Build history of the part. All positions in model axes, mm. Face numbers are marked on the shaded views. Give positions to 0.01 mm unless a question says otherwise; leave off trailing zeros. Order: outer loops, then holes, each group sorted by start corner. A loop starts at its lowest first (then second) coordinate and runs counter-clockwise, first axis right, second up. Notation, with made-up numbers: M 59,71 L 96,71 A18 cw 96,100 Z; hole C -34,72 d10. An arc over 180 degrees is marked long. Answer as CSV lines item,"result".
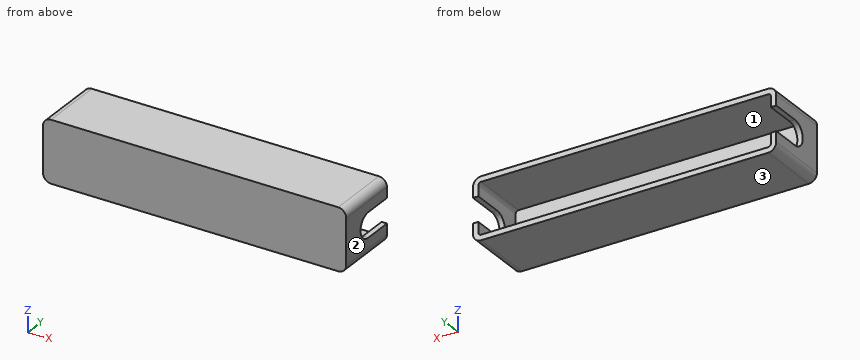
from build123d import *

# Parameters (mm, degrees)
BOSS_EXTRUDE1_DEPTH = 24
SHELL2_T            = -2
CUT_EXTRUDE1_DEPTH  = 117.091558694


with BuildPart() as part:
    # Sketch1 → Boss-Extrude1 (new body)
    with BuildSketch(Plane(origin=(0, 0, 0), x_dir=(1, 0, 0), z_dir=(0, 1, 0))):
        with BuildLine():
            Line((-53.5, -11.5), (53.5, -11.5))
            ThreePointArc((53.5, -11.5), (55.621320344, -10.621320344), (56.5, -8.5))
            Line((56.5, -8.5), (56.5, 8.5))
            ThreePointArc((56.5, 8.5), (55.621320344, 10.621320344), (53.5, 11.5))
            Line((53.5, 11.5), (-53.5, 11.5))
            ThreePointArc((-53.5, 11.5), (-55.621320344, 10.621320344), (-56.5, 8.5))
            Line((-56.5, 8.5), (-56.5, -8.5))
            ThreePointArc((-56.5, -8.5), (-55.621320344, -10.621320344), (-53.5, -11.5))
        make_face()
    extrude(amount=BOSS_EXTRUDE1_DEPTH)

    # Shell2
    shell2_openings = [part.faces().sort_by_distance(p)[0] for p in [
        (0, 24, 0),
    ]]
    offset(amount=SHELL2_T, openings=shell2_openings, kind=Kind.INTERSECTION)

    # Sketch4 → Cut-Extrude1 (cut, through all)
    with BuildSketch(Plane(origin=(56.5, 0, 0), x_dir=(0, 0, -1), z_dir=(1, 0, 0))):
        with BuildLine():
            Line((-4.588804417, 24), (-4.588804417, 13))
            ThreePointArc((-4.588804417, 13), (0, 8.411195583), (4.588804417, 13))
            Line((4.588804417, 13), (4.588804417, 24))
            Line((4.588804417, 24), (-4.588804417, 24))
        make_face()
    extrude(amount=-CUT_EXTRUDE1_DEPTH, mode=Mode.SUBTRACT)


solid = part.part
Item 1: Band-saw the part on A-A (y = 17). Give the cut face in (x, z).
Geometry says:
outline,"M -56.5,-8.5 A3 ccw -53.5,-11.5 L 53.5,-11.5 A3 ccw 56.5,-8.5 L 56.5,-4.59 L 54.5,-4.59 L 54.5,-8.5 A1 cw 53.5,-9.5 L -53.5,-9.5 A1 cw -54.5,-8.5 L -54.5,-4.59 L -56.5,-4.59 Z; M -56.5,4.59 L -54.5,4.59 L -54.5,8.5 A1 cw -53.5,9.5 L 53.5,9.5 A1 cw 54.5,8.5 L 54.5,4.59 L 56.5,4.59 L 56.5,8.5 A3 ccw 53.5,11.5 L -53.5,11.5 A3 ccw -56.5,8.5 Z"
Item 2: Band-saw the part on B-B (x = 14.5). Give the cut face in (y, z).
Geometry says:
outline,"M 0,-11.5 L 24,-11.5 L 24,-9.5 L 2,-9.5 L 2,9.5 L 24,9.5 L 24,11.5 L 0,11.5 Z"
Item 3: Band-saw the part on D-D (y = 10). Give the cut face in (x, z), and give its area (3 significant figures).
Geometry says:
outline,"M -56.5,-8.5 A3 ccw -53.5,-11.5 L 53.5,-11.5 A3 ccw 56.5,-8.5 L 56.5,-3.47 L 54.5,-3.47 L 54.5,-8.5 A1 cw 53.5,-9.5 L -53.5,-9.5 A1 cw -54.5,-8.5 L -54.5,-3.47 L -56.5,-3.47 Z; M -56.5,3.47 L -54.5,3.47 L -54.5,8.5 A1 cw -53.5,9.5 L 53.5,9.5 A1 cw 54.5,8.5 L 54.5,3.47 L 56.5,3.47 L 56.5,8.5 A3 ccw 53.5,11.5 L -53.5,11.5 A3 ccw -56.5,8.5 Z"
area,"493 mm2"
Item 4: Probe line 1 along X through (y, z) = (17, 7.25); line 2 along Z through (x, y) = (36, 13); line 3 along Y through (x, z) = (40.5, 8). List the from-to ranges inside material, lowest first. Write a range as from..to.
Geometry says:
line 1,"x = -56.5..-54.5, 54.5..56.5"
line 2,"z = -11.5..-9.5, 9.5..11.5"
line 3,"y = 0..2"
Item 5: Drop flat-ended pins along their axis: pin 1 (2 mm diameter, centred on x = 55, y = 17.5, fed in from +Z); pin 2 (0.6 mm diameter, centred on x = -56, y = 20, fed in from +Z); pin 3 (1.6 mm diameter, centred on x = 55.5, y = 18.5, fed in from -Z). Give the stop position or say it passes through.
Geometry says:
pin 1,"stops at z = 11.46"
pin 2,"stops at z = 10.54"
pin 3,"stops at z = -11.25"
Item 6: Band-saw the part on C-C (z = 0). Give the cut face in (x, y).
Geometry says:
outline,"M -56.5,0 L 56.5,0 L 56.5,8.41 L 54.5,8.41 L 54.5,2 L -54.5,2 L -54.5,8.41 L -56.5,8.41 Z"
Item 7: Pull direction Z, two halves, no side cores. Call the marked faces 1, 2 and 3: released by +Z, released by -Z, zero draft, split by the parting line, or undercut.
Geometry says:
face 1,"undercut"
face 2,"zero draft"
face 3,"released by -Z"
